Geometry check sheet. Reference: drawing and pictorial views, mm from the part's lowest x, y, z. A direction names the side the tool comes from. Round coordinates to 2 decimals unless told otherwise and drop trailing zeros. Order: outer loops, then holes, each group sorted by start corner. A loop starts at its lowest first (then second) coordinate and runs counter-clockwise, first axis right, second up.
(1) Draft check along X on the marked faces 1, 2, 3 and 4. Enter one of: pulls with the +X half, pulls with the -X half, needs draft (parallel to the pull), parting line crosses it, or undercut.
(2) Thickness scan on L1, parallel to Z at x = 10.5, y = 2.8; L2, parallel to Z at x = 13.25, y = 4.3; L3, parallel to Z at x = 10.25, y = 5.1. Record the ranges inside material, lowest first.
(3) Cross-section at C-C on z = 3.5. Enter the section's corners in (x, y), and give its area (3 significant figures).
(4) Cross-section at D-D on z = 11. Enter the section's corners in (x, y), and give its area (3 significant figures).
(5) Set-up check for the marked faces 5, 6 and 7: record each of +Z, -Z, +X, -X, +Y, -Y from which the full face is reachable in a straight line by a thin tool's end or side.
(6) Cross-section at B-B on y = 4.5. Count the separate pieces of the cut face and the enclosed holes in it, and give its area (3 significant figures).
(7) Cross-section at A-A on x = 3.5. Enter the section's corners in (y, z), and give its area (3 significant figures).
(8) Gauge pin test, flat ends, axial feed: P1, Ø1.3, axis at x = 3.035, z = 7.755, coming from the +Y side; P2, Ø1, axis at x = 10.5, z = 12, coming from the -Y side; P3, Ø2, axis at y = 3.5, z = 13.5, coming from the +X side; P4, Ø1.5, axis at x = 9, y = 2, coming from the +Z side. Record the tip position at first contact, or that the pin passes through.
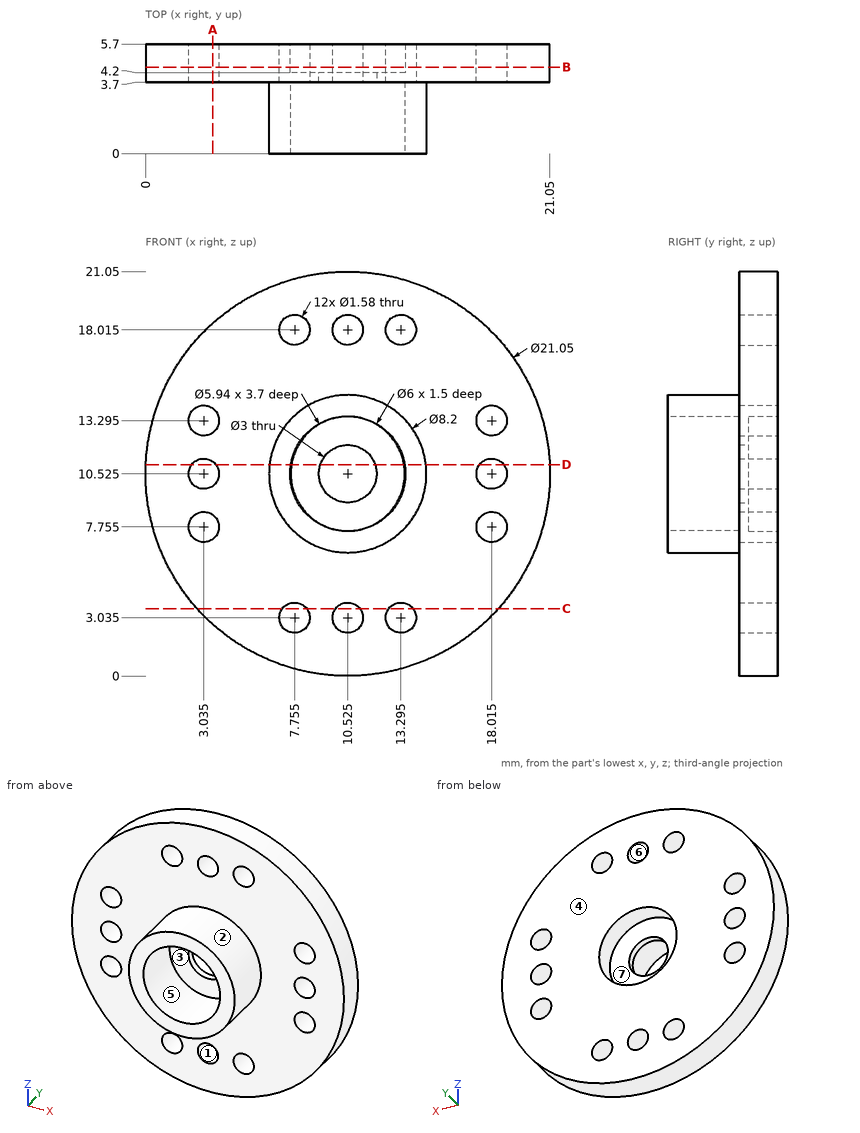
Found:
1. face 1: undercut
1. face 2: parting line crosses it
1. face 3: undercut
1. face 4: needs draft
2. L1: z = 6.43 to 7.56, 13.49 to 14.62
2. L2: z = 0.36 to 2.25, 3.82 to 9.27, 11.78 to 17.23, 18.8 to 20.69
2. L3: z = 0 to 2.29, 3.78 to 7.54, 13.51 to 17.27, 18.76 to 21.05
3. outline: (2.69, 3.7) - (7.12, 3.7) - (7.12, 5.7) - (2.69, 5.7) - close; (8.39, 3.7) - (9.89, 3.7) - (9.89, 5.7) - (8.39, 5.7) - close; (11.16, 3.7) - (12.66, 3.7) - (12.66, 5.7) - (11.16, 5.7) - close; (13.93, 3.7) - (18.36, 3.7) - (18.36, 5.7) - (13.93, 5.7) - close
3. area: 23.7 mm2
4. outline: (0.01, 3.7) - (2.4, 3.7) - (2.4, 5.7) - (0.01, 5.7) - close; (3.67, 3.7) - (6.45, 3.7) - (6.45, 0) - (7.59, 0) - (7.59, 3.7) - (9.1, 3.7) - (9.1, 4.2) - (7.56, 4.2) - (7.56, 5.7) - (3.67, 5.7) - close; (11.95, 3.7) - (13.46, 3.7) - (13.46, 0) - (14.6, 0) - (14.6, 3.7) - (17.38, 3.7) - (17.38, 5.7) - (13.49, 5.7) - (13.49, 4.2) - (11.95, 4.2) - close; (18.65, 3.7) - (21.04, 3.7) - (21.04, 5.7) - (18.65, 5.7) - close
4. area: 35.1 mm2
5. face 5: -Y
5. face 6: +Y, -Y
5. face 7: +Y
6. separate pieces: 1
6. enclosed holes: 13
6. area: 296 mm2
7. outline: (3.7, 2.69) - (5.7, 2.69) - (5.7, 7.12) - (3.7, 7.12) - close; (3.7, 8.39) - (5.7, 8.39) - (5.7, 9.89) - (3.7, 9.89) - close; (3.7, 11.16) - (5.7, 11.16) - (5.7, 12.66) - (3.7, 12.66) - close; (3.7, 13.93) - (5.7, 13.93) - (5.7, 18.36) - (3.7, 18.36) - close
7. area: 23.7 mm2
8. P1: passes through
8. P2: stops at y = 3.7
8. P3: stops at x = 20.86
8. P4: stops at z = 14.55
